from build123d import *

# Parameters (mm, degrees)
SKETCH2_R           = 1.5
SKETCH2_W           = 3
SKETCH2_H           = 10
BOSS_EXTRUDE2_DEPTH = 5
CUT_EXTRUDE1_DEPTH  = 6


with BuildPart() as part:
    # Sketch2 → Boss-Extrude2 (new body)
    with BuildSketch(Plane(origin=(0, 0, 0), x_dir=(1, 0, 0), z_dir=(0, 1, 0))):
        Polygon((9.607122403, -57.726350335), (39.607122403, -57.726350335), (39.607122403, -40.226350335), (46.607122403, -40.226350335), (46.607122403, -18.226350335), (39.607122403, -18.226350335), (39.607122403, -3.226350335), (9.607122403, -3.226350335), (9.607122403, -18.226350335), (2.607122403, -18.226350335), (2.607122403, -40.226350335), (9.607122403, -40.226350335), align=None)
        with Locations((41.607122403, -22.726350335)):
            Circle(SKETCH2_R, mode=Mode.SUBTRACT)
        with Locations((41.607122403, -35.726350335)):
            Circle(SKETCH2_R, mode=Mode.SUBTRACT)
        with Locations((7.607122403, -35.726350335)):
            Circle(SKETCH2_R, mode=Mode.SUBTRACT)
        with Locations((7.607122403, -22.726350335)):
            Circle(SKETCH2_R, mode=Mode.SUBTRACT)
        with Locations((33.107122403, -29.226350335)):
            Rectangle(SKETCH2_W, SKETCH2_H, mode=Mode.SUBTRACT)
        with Locations((16.107122403, -29.226350335)):
            Rectangle(SKETCH2_W, SKETCH2_H, mode=Mode.SUBTRACT)
    extrude(amount=BOSS_EXTRUDE2_DEPTH)

    # Sketch3 → Cut-Extrude1 (cut, through all)
    with BuildSketch(Plane(origin=(0, 5, 0), x_dir=(-1, 0, 0), z_dir=(0, 1, 0))):
        Polygon((-39.607122403, 46.526350335), (-35.607122403, 46.526350335), (-35.607122403, 44.976350335), (-33.407122403, 44.976350335), (-33.407122403, 46.526350335), (-31.407122403, 46.526350335), (-31.407122403, 48.926350335), (-33.407122403, 48.926350335), (-33.407122403, 50.476350335), (-35.607122403, 50.476350335), (-35.607122403, 48.926350335), (-39.607122403, 48.926350335), align=None)
        Polygon((-39.607122403, 9.526350335), (-35.607122403, 9.526350335), (-35.607122403, 7.976350335), (-33.407122403, 7.976350335), (-33.407122403, 9.526350335), (-31.407122403, 9.526350335), (-31.407122403, 11.926350335), (-33.407122403, 11.926350335), (-33.407122403, 13.476350335), (-35.607122403, 13.476350335), (-35.607122403, 11.926350335), (-39.607122403, 11.926350335), align=None)
        Polygon((-13.607122403, 50.476350335), (-15.807122403, 50.476350335), (-15.807122403, 48.926350335), (-17.807122403, 48.926350335), (-17.807122403, 46.526350335), (-15.807122403, 46.526350335), (-15.807122403, 44.976350335), (-13.607122403, 44.976350335), (-13.607122403, 46.526350335), (-9.607122403, 46.526350335), (-9.607122403, 48.926350335), (-13.607122403, 48.926350335), align=None)
        Polygon((-9.607122403, 11.926350335), (-13.607122403, 11.926350335), (-13.607122403, 13.476350335), (-15.807122403, 13.476350335), (-15.807122403, 11.926350335), (-17.807122403, 11.926350335), (-17.807122403, 9.526350335), (-15.807122403, 9.526350335), (-15.807122403, 7.976350335), (-13.607122403, 7.976350335), (-13.607122403, 9.526350335), (-9.607122403, 9.526350335), align=None)
    extrude(amount=-CUT_EXTRUDE1_DEPTH, mode=Mode.SUBTRACT)


solid = part.part
Could you check a few things on this model? Use its own coordinates, in mm. A direction names the side the tool comes from. Coordinates: 2 decimals unless noted, no trailing zeros. Loops run counter-clockwise (first coordinate to the right, second up) from the corner with the lowest first, then second, coordinate; pieces in that order, holes last.
1. Imagine slicing it at C-C (z = 23.5). Please give me the cut outline in (x, y).
2. For P1, Ø0.5, axis at y = 2, z = 12.5, coming from the -X side; P2, Ø1.5, axis at x = 6.5, y = 3, coming from the -Z side; P3, Ø0.7, axis at y = 2, z = 48, coming from the -X side, each with a flat end and sliding along its axis, tell me the tip position at first contact or that it passes through.
3. I need wall thicknesses on L1, parallel to Z at x = 12.5, y = 3.25; L2, parallel to X at y = 0.55, z = 31; L3, parallel to X at y = 2.35, z = 46. Which ranges of each line are inside material? Lowest first, please.
4. Imagine slicing it at D-D (y = 4.15). Give the number of separate pieces and of enclosed holes in the cut face, and give its area (3 significant figures).
5. Imagine slicing it at A-A (x = 17). Please give me the cut outline in (y, z).
6. Imagine slicing it at B-B (x = 36.5). Please give me the cut outline in (y, z).
7. For faces 4 (the face through (6, 2, 40.226)), 5 (the face through (13.607, 3, 50)), 6 (the face through (32, 3, 9.526)), 7 (the face through (17.807, 3, 11)), which set-ups out of +Z, -Z, +X, -X, +Y, -Y let a thin tool reach every point of the face, with its end or its side?
8. We'd pull the mould along X, two halves only. Please class faces 1 (the face through (39.607, 2, 6)), 2 (the face through (17.807, 3, 48)), 3 (the face through (35, 3, 44.976)): released by +X, released by -X, zero draft, split by the parting line, or undercut.
Computed values:
1. outline: (2.61, 0) - (6.32, 0) - (6.32, 5) - (2.61, 5) - close; (8.89, 0) - (40.32, 0) - (40.32, 5) - (8.89, 5) - close; (42.89, 0) - (46.61, 0) - (46.61, 5) - (42.89, 5) - close
2. P1: stops at x = 9.61
2. P2: stops at z = 18.23
2. P3: stops at x = 17.81
3. L1: z = 3.23 to 9.53, 11.93 to 46.53, 48.93 to 57.73
3. L2: x = 2.61 to 14.61, 17.61 to 31.61, 34.61 to 46.61
3. L3: x = 9.61 to 13.61, 15.81 to 33.41, 35.61 to 39.61
4. separate pieces: 1
4. enclosed holes: 6
4. area: 1,750 mm2
5. outline: (0, 3.23) - (5, 3.23) - (5, 9.53) - (0, 9.53) - close; (0, 11.93) - (5, 11.93) - (5, 24.23) - (0, 24.23) - close; (0, 34.23) - (5, 34.23) - (5, 46.53) - (0, 46.53) - close; (0, 48.93) - (5, 48.93) - (5, 57.73) - (0, 57.73) - close
6. outline: (0, 3.23) - (5, 3.23) - (5, 9.53) - (0, 9.53) - close; (0, 11.93) - (5, 11.93) - (5, 46.53) - (0, 46.53) - close; (0, 48.93) - (5, 48.93) - (5, 57.73) - (0, 57.73) - close
7. face 4: +Z, -X, +Y, -Y
7. face 5: +Y, -Y
7. face 6: +X, +Y, -Y
7. face 7: -X, +Y, -Y
8. face 1: released by +X
8. face 2: released by -X
8. face 3: undercut
